Autodesk Inventor part; units mm, degrees
ref_plane "YZ Plane" through (0, 0, 0) normal (1, 0, 0) x (0, 1, 0)
ref_plane "XZ Plane" through (0, 0, 0) normal (0, 1, 0) x (-1, 0, 0)
ref_plane "XY Plane" through (0, 0, 0) normal (0, 0, 1) x (1, 0, 0)
sketch "Sketch1" plane through (0, 0, 0) normal (0, 0, 1) x (1, 0, 0)
  line L0 (-24.5, 26) -> (24.5, 26)
  line L1 (24.5, 26) -> (24.5, -26)
  line L2 (24.5, -26) -> (-24.5, -26)
  line L3 (-24.5, -26) -> (-24.5, 26)
  point P0 (0, 0)
  dimension "d0" = 52
  dimension "d1" = 26
  dimension "d2" = 49
  dimension "d3" = 24.5
extrude "Extrusion1" add sketch "Sketch1" along normal blind 11.05
sketch "Sketch3" plane through (0, 0, 11.05) normal (0, 0, 1) x (1, 0, 0)
  line L0 (-24.5, -26) -> (24.5, -26)
  line L1 (0, -26) -> (0, -20.5)
  line L2 (24.5, 26) -> (-24.5, 26)
  line L3 (0, 26) -> (0, 20.5)
  point P0 (0, 0)
  point P1 (0, 0)
  dimension "d13" = 5.5
  dimension "d14" = 20.5
  dimension "d15" = 5.5
  dimension "d16" = 20.5
hole "Hole1" at (0, 20.5, 11.05) at (0, -20.5, 11.05) direction (0, 0, -1) diameter 4.305 depth 12.3 counterbore diameter 7.938 counterbore depth 2.4
fillet "Fillet1" radius 2 4 edges at (-24.5, -26, 5.525) (-24.5, 26, 5.525) (24.5, -26, 5.525) (24.5, 26, 5.525)
sketch "Sketch7" plane through (-24.5, -24, 0) normal (-1, 0, 0) x (0, 0, 1)
  circle A0 centre (-12.35, 24) radius 12.7
  point P0 (0, 24)
  dimension "d57" = 25.4
  dimension "d58" = 12.35
extrude "Extrusion3" cut sketch "Sketch7" against normal blind 50
sketch "Sketch11" plane through (0, 0, 11.05) normal (0, 0, 1) x (1, 0, 0)
  line L0 (0, 0) -> (0, -15) construction
  line L1 (0, 0) -> (0, 15) construction
  line L2 (0, 0) -> (22.5, 0) construction
  line L3 (22.5, 0) -> (22.5, -15) construction
  line L4 (22.5, 0) -> (22.5, 15) construction
  line L5 (0, 0) -> (-22.5, 0) construction
  line L6 (-22.5, 0) -> (-22.5, -15) construction
  line L7 (-22.5, 0) -> (-22.5, 15) construction
  line L8 (22.5, -15) -> (-22.5, -15) construction
  line L9 (22.5, 15) -> (-22.5, 15) construction
  line L10 (-15.4375, 7.9375) -> (15.4375, 7.9375) construction
  line L11 (15.4375, -7.9375) -> (-15.4375, -7.9375) construction
  line L12 (-18.6125, -11.1125) -> (-18.6125, 0) construction
  line L13 (-18.6125, 0) -> (-18.6125, 11.1125) construction
  line L14 (18.6125, 11.1125) -> (18.6125, 0) construction
  line L15 (18.6125, 0) -> (18.6125, -11.1125) construction
  line L16 (15.4375, -7.9375) -> (18.6125, -7.9375) construction
  line L17 (15.4375, 7.9375) -> (18.6125, 7.9375) construction
  line L18 (-15.4375, -7.9375) -> (-18.6125, -7.9375) construction
  line L19 (-15.4375, 7.9375) -> (-18.6125, 7.9375) construction
  line L20 (18.6125, -7.9375) -> (29.1538, -7.9375) construction
  line L21 (18.6125, 7.9375) -> (28.0959, 7.9375) construction
  line L22 (-18.6125, -7.9375) -> (-33.3375, -7.9375) construction
  line L23 (-18.6125, 7.9375) -> (-34.925, 7.9375) construction
  dimension "d98" = 22.5
  dimension "d99" = 15
  dimension "d100" = 15
  dimension "d101" = 22.5
  dimension "d102" = 15
  dimension "d103" = 15
  dimension "d104" = 7.0625
hole "Hole6" [suppressed]
sketch "Sketch12" plane through (0, 0, 0) normal (0, 0, -1) x (-1, 0, 0)
  line L0 (-22.5, 0) -> (-22.5, 15) construction
  line L1 (22.5, 0) -> (22.5, 15) construction
  line L2 (-22.5, 0) -> (-22.5, -15) construction
  line L3 (22.5, 0) -> (22.5, -15) construction
  line L4 (24.5, 24) -> (24.5, -24) construction
  line L5 (-22.5, 15) -> (22.5, 15) construction
  line L6 (-22.5, -15) -> (22.5, -15) construction
  line L7 (-18.5, 11.55) -> (-18.5, 0) construction
  line L8 (-18.5, 0) -> (-18.5, -11.55) construction
  line L9 (18.5, -11.55) -> (18.5, 0) construction
  line L10 (18.5, 0) -> (18.5, 11.55) construction
  line L11 (15.9875, -7.5) -> (-14.8875, -7.5) construction
  line L12 (-15.4375, 7.5) -> (15.4375, 7.5) construction
  line L13 (-15.4375, 7.5) -> (-18.5, 7.5) construction
  line L14 (15.4375, 7.5) -> (18.5, 7.5) construction
  line L15 (-14.8875, -7.5) -> (-18.5, -7.5) construction
  line L16 (15.9875, -7.5) -> (18.5, -7.5) construction
  line L17 (-18.5, 7.5) -> (-21.7329, 7.5) construction
  line L18 (-18.5, -7.5) -> (-20.6685, -7.5) construction
  line L19 (18.5, -7.5) -> (22.1748, -7.5) construction
  line L20 (18.5, 7.5) -> (20.6375, 7.5) construction
  point P0 (0, 0)
  dimension "d115" = 15
  dimension "d117" = 4
  dimension "d118" = 7.5
  dimension "d126" = 45
  dimension "d127" = 15
  dimension "d128" = 4
  dimension "d129" = 7.5
hole "Hole7" at (18.5, 7.5, 0) at (-18.5, 7.5, 0) at (18.5, -7.5, 0) at (-18.5, -7.5, 0) direction (0, 0, 1) diameter 2.9 end through all counterbore diameter 5.5 counterbore depth 2.5
equation "\"d15\" = d13"
properties part number "ADAPTER_EOM2.1GHz_new"
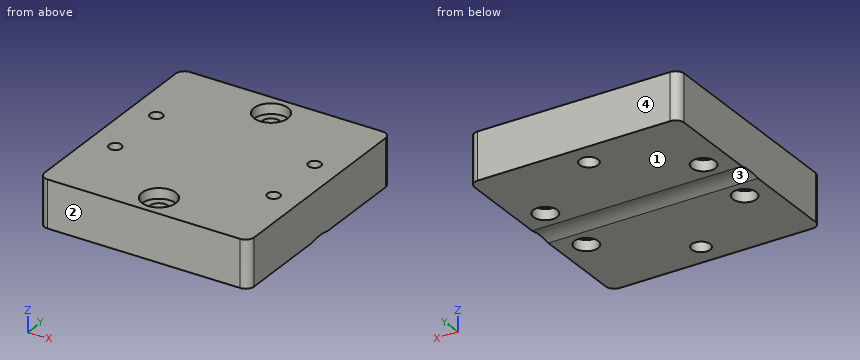
Input: part model. Units: mm. Frame: model coordinates. Face numbers are marked on the shaded views. Give positions to 0.01 mm unless a question says otherwise; leave off trailing zeros. Loops run counter-clockwise (first coordinate to the right, second up) from the corner with the lowest first, then second, coordinate; pieces in that order, holes last. Notation, with made-up numbers: (14.25, 66) -> (25.25, 66) arc R28 cw to (25.25, 94) -> close; hole circle Ø11 at (21, 10). An arc over 180 degrees is marked (long way). Use a Markdown table: item, result.
Q1. Section query B-B, the plane y = -20.5. Return the cut outline in (x, z), plus the area to 3 significant figures.
Entries:
| item | result |
|---|---|
| outline | (-24.5, 0) -> (-2.15, 0) -> (-2.15, 8.65) -> (-3.97, 8.65) -> (-3.97, 11.05) -> (-24.5, 11.05) -> close; (2.15, 0) -> (24.5, 0) -> (24.5, 11.05) -> (3.97, 11.05) -> (3.97, 8.65) -> (2.15, 8.65) -> close |
| area | 485 mm² |
Q2. Section query C-C, the plane z = 1.75. State how many separate pieces and enclosed holes the cut face has, plus the area to 3 significant figures.
Entries:
| item | result |
|---|---|
| separate pieces | 1 |
| enclosed holes | 6 |
| area | 2,420 mm² |
Q3. Section query A-A, the plane x = 0. Return the cut outline in (y, z), plus the area to 3 significant figures.
Entries:
| item | result |
|---|---|
| outline | (-26, 0) -> (-22.65, 0) -> (-22.65, 8.65) -> (-24.47, 8.65) -> (-24.47, 11.05) -> (-26, 11.05) -> close; (-18.35, 0) -> (-2.96, 0) arc R12.7 cw to (2.96, 0) -> (18.35, 0) -> (18.35, 8.65) -> (16.53, 8.65) -> (16.53, 11.05) -> (-16.53, 11.05) -> (-16.53, 8.65) -> (-18.35, 8.65) -> close; (22.65, 0) -> (26, 0) -> (26, 11.05) -> (24.47, 11.05) -> (24.47, 8.65) -> (22.65, 8.65) -> close |
| area | 461 mm² |
Q4. First-contact query: P1, Ø2.5, axis at x = -0.5, y = 22.5, coming from the +Z side; P2, Ø3, axis at x = -19, y = 8, coming from the -Z side. Flat tips, straight axial feed; report the tip coordinate or a pass-through.
Entries:
| item | result |
|---|---|
| P1 | stops at z = 8.65 |
| P2 | stops at z = 2.5 |
Q5. Pull-direction query (Y, two-part tool) for the marked faces 1, 2, 3 and 4; classes: pulls with the +Y half, pulls with the -Y half, needs draft (parallel to the pull), parting line crosses it, or undercut.
Entries:
| item | result |
|---|---|
| face 1 | needs draft |
| face 2 | pulls with the -Y half |
| face 3 | undercut |
| face 4 | pulls with the +Y half |
Q6. Section query D-D, the plane y = 7.5. Return the cut outline in (x, z), plus the area to 3 significant figures.
Entries:
| item | result |
|---|---|
| outline | (-24.5, 0) -> (-21.25, 0) -> (-21.25, 2.5) -> (-19.95, 2.5) -> (-19.95, 11.05) -> (-24.5, 11.05) -> close; (-17.05, 2.5) -> (-15.75, 2.5) -> (-15.75, 0) -> (15.75, 0) -> (15.75, 2.5) -> (17.05, 2.5) -> (17.05, 11.05) -> (-17.05, 11.05) -> close; (19.95, 2.5) -> (21.25, 2.5) -> (21.25, 0) -> (24.5, 0) -> (24.5, 11.05) -> (19.95, 11.05) -> close |
| area | 464 mm² |
Q7. Ray query, probe 1 along Y at (x, z) = (-18.5, 0.6); probe 2 along Y at (x, z) = (0, 9.75); probe 3 along X at (y, z) = (7.5, 0.75). Return the intervals inside material, ascending. Write a range as from..to.
Entries:
| item | result |
|---|---|
| probe 1 | y = -26..-10.25, -4.75..4.75, 10.25..26 |
| probe 2 | y = -26..-24.47, -16.53..16.53, 24.47..26 |
| probe 3 | x = -24.5..-21.25, -15.75..15.75, 21.25..24.5 |
